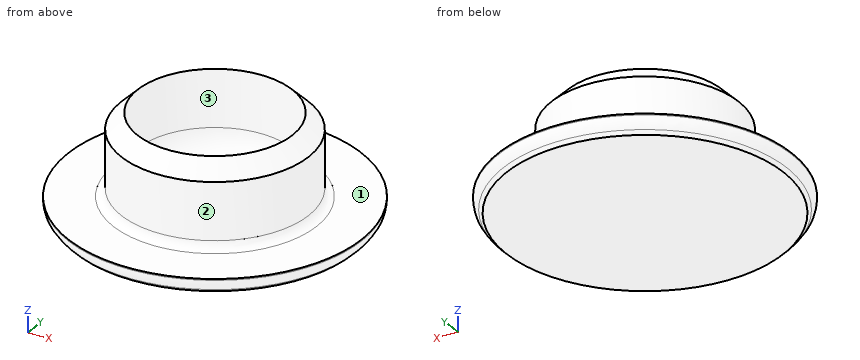
from build123d import *

# Parameters (mm, degrees)
F2_R = 3
F3_R = 2
F4_R = 1


with BuildPart() as f1:
    # F0 (on Front) → F1 (revolve)
    with BuildSketch(Plane.XZ):
        Polygon((0, 2), (0, 0), (17, 0), (18, 1), (18, 2), (11.5, 2), (11.5, 10), (9.5, 12), (9.5, 2), align=None)
    revolve(axis=Axis((0, 0, 1), (0, 0, -1)))

    # F2
    f2_edges = [f1.edges().sort_by_distance(p)[0] for p in [
        (-9.5, 0, 2),
    ]]
    fillet(f2_edges, radius=F2_R)

    # F3
    f3_edges = [f1.edges().sort_by_distance(p)[0] for p in [
        (-18, 0, 1),
    ]]
    fillet(f3_edges, radius=F3_R)

    # F4
    f4_edges = [f1.edges().sort_by_distance(p)[0] for p in [
        (-11.5, 0, 2),
    ]]
    fillet(f4_edges, radius=F4_R)


solid = f1.part
CAD build for the part. Positions are in the model's coordinates, mm. Face numbers are marked on the shaded views. Round coordinates to 2 decimals unless told otherwise and drop trailing zeros. Loops run counter-clockwise (first coordinate to the right, second up) from the corner with the lowest first, then second, coordinate; pieces in that order, holes last.
(1) Cut at A-A (z = 11.5). Give the cut face in (x, y), plus the area to 3 significant figures.
(2) Two-plate mould, pull along X, no slides. Class the marked faces 1, 2 and 3: +X half, -X half, draft (parallel to the pull), parting line (faces both ways), or undercut.
(3) Cut at B-B (z = 8.5). Give the cut face in (x, y).
(4) Wall check: line 1 along X through (y, z) = (0, 10); line 2 along X through (y, z) = (-0.5, 4). Give the ranges that are in metal, low to high.
(5) Drop flat-ended pins along their axis: pin 1 (1.5 mm diameter, centred on y = 1.5, z = 5.5, fed in from +X); pin 2 (4 mm diameter, centred on x = 3.5, z = 8.5, fed in from -Y); pin 3 (4 mm diameter, centred on x = -0.5, z = 10, fed in from -Y). Give the stop position or say it passes through.
Findings below:
1. outline: circle Ø20 at (0, 0); hole circle Ø19 at (0, 0)
1. area: 30.6 mm2
2. face 1: draft
2. face 2: parting line
2. face 3: undercut
3. outline: circle Ø23 at (0, 0); hole circle Ø19 at (0, 0)
4. line 1: x = -11.5 to -9.5, 9.5 to 11.5
4. line 2: x = -11.49 to -9.32, 9.32 to 11.49
5. pin 1: stops at x = 11.48
5. pin 2: stops at y = -11.4
5. pin 3: stops at y = -11.5
